from build123d import *

# Parameters (mm, degrees)
SKETCH1_R           = 5.9375
SKETCH1_R_2         = 1.4375
BOSS_EXTRUDE1_DEPTH = 6.35
SKETCH8_R           = 1.5
CUT_EXTRUDE1_DEPTH  = 45.18177233


with BuildPart() as part:
    # Sketch1 → Boss-Extrude1 (new body)
    with BuildSketch(Plane.XY):
        with BuildLine():
            ThreePointArc((7.766045394, -32.993333104), (18.228763262, -27.492050685), (19.627171546, -15.754204728))
            Line((19.627171546, -15.754204728), (11.861126152, 4.539128375))
            ThreePointArc((11.861126152, 4.539128375), (1.909586496, 12.555615453), (-9.975303898, 7.860236137))
            Line((-9.975303898, 7.860236137), (-25.965833293, -12.433096966))
            ThreePointArc((-25.965833293, -12.433096966), (-27.416705459, -25.837023258), (-15.990529394, -32.993333104))
            Line((-15.990529394, -32.993333104), (7.766045394, -32.993333104))
        make_face()
        with Locations((-15.990529394, -20.293333104)):
            Circle(SKETCH1_R, mode=Mode.SUBTRACT)
        with Locations((7.766045394, -20.293333104)):
            Circle(SKETCH1_R, mode=Mode.SUBTRACT)
        Circle(SKETCH1_R_2, mode=Mode.SUBTRACT)
    extrude(amount=BOSS_EXTRUDE1_DEPTH)

    # Sketch8 → Cut-Extrude1 (cut, through all)
    with BuildSketch(Plane.XY.offset(6.35)):
        with Locations((7.766045394, -10.768333104)):
            Circle(SKETCH8_R)
        with Locations((-15.990529394, -29.818333104)):
            Circle(SKETCH8_R)
        with Locations((-24.239421365, -15.530833104)):
            Circle(SKETCH8_R)
        with Locations((-7.741637423, -15.530833104)):
            Circle(SKETCH8_R)
        with Locations((16.014937365, -25.055833104)):
            Circle(SKETCH8_R)
        with Locations((-0.482846577, -25.055833104)):
            Circle(SKETCH8_R)
    extrude(amount=-CUT_EXTRUDE1_DEPTH, mode=Mode.SUBTRACT)


solid = part.part
The model under review builds one solid part; all positions refer to its coordinate system, in mm. Coordinates: 2 decimals unless noted, no trailing zeros. Write each loop counter-clockwise with the first axis right and the second up, starting at its lowest first coordinate (ties: lowest second). Pieces come first, ordered by that corner, then holes. Notation, with made-up numbers: (-15.75, 50.5) -> (17.25, 50.5) arc R16 cw to (17.25, 63.5) -> close; hole circle Ø6 at (8.5, 77.5). An arc over 180 degrees is marked (long way). Answer in a Markdown table with one row per item.
1. Clearance check with flat-ended pins moving along their axes: pin 1 Ø10.5 at (x, y) = (-15.99, -20.29) entering from +Z; pin 2 Ø3 at (y, z) = (-2.5, 3) entering from -X. State where each tip first meets the part, or that it passes through.
Answers below:
| item | result |
|---|---|
| pin 1 | passes through |
| pin 2 | stops at x = -19.32 |
2. Draft analysis for pull direction X (two halves, no side actions). For faces 1 (the flat face through (15.8, -5.75, 3.13)), 2 (the cylindrical face through (15.69, -26.52, 3.22)), 3 (the cylindrical face through (-0.81, -26.52, 3.22)), 4 (the cylindrical face through (2.095, 12.526, 3.131)), state which applies: +X half, -X half, draft (parallel to the pull), parting line (faces both ways), or undercut.
Answers below:
| item | result |
|---|---|
| face 1 | +X half |
| face 2 | undercut |
| face 3 | undercut |
| face 4 | parting line |
3. We need section A-A, the plane x = 10. State the section outline as (y, z) points, and give its area (3 significant figures).
Answers below:
| item | result |
|---|---|
| outline | (-32.8, 0) -> (-25.79, 0) -> (-25.79, 6.35) -> (-32.8, 6.35) -> close; (-14.79, 0) -> (7.83, 0) -> (7.83, 6.35) -> (-14.79, 6.35) -> close |
| area | 188 mm^2 |
4. We need section C-C, the plane x = 0. State the section outline as (y, z) points, and give its area (3 significant figures).
Answers below:
| item | result |
|---|---|
| outline | (-32.99, 0) -> (-26.48, 0) -> (-26.48, 6.35) -> (-32.99, 6.35) -> close; (-23.64, 0) -> (-1.44, 0) -> (-1.44, 6.35) -> (-23.64, 6.35) -> close; (1.44, 0) -> (12.7, 0) -> (12.7, 6.35) -> (1.44, 6.35) -> close |
| area | 254 mm^2 |
5. We need section B-B, the plane y = 0. State the section outline as (x, z) points, and give its area (3 significant figures).
Answers below:
| item | result |
|---|---|
| outline | (-16.17, 0) -> (-1.44, 0) -> (-1.44, 6.35) -> (-16.17, 6.35) -> close; (1.44, 0) -> (13.6, 0) -> (13.6, 6.35) -> (1.44, 6.35) -> close |
| area | 171 mm^2 |
6. We need section D-D, the plane y = -18. State the section outline as (x, z) points.
Answers below:
| item | result |
|---|---|
| outline | (-28.48, 0) -> (-21.47, 0) -> (-21.47, 6.35) -> (-28.48, 6.35) -> close; (-10.51, 0) -> (2.29, 0) -> (2.29, 6.35) -> (-10.51, 6.35) -> close; (13.24, 0) -> (20.26, 0) -> (20.26, 6.35) -> (13.24, 6.35) -> close |
7. Wall thickness on probe 1 along X at (y, z) = (-15, 4.75); probe 2 along Y at (x, z) = (0, 2.25); probe 3 along X at (y, z) = (-18, 2.5): over which ranges is each line inside the solid? List them lowest first. Write a range as [from, to].
Answers below:
| item | result |
|---|---|
| probe 1 | x = [-27.53, -25.64], [-22.84, -18.68], [-13.3, -9.14], [-6.34, 5.08], [10.46, 19.34] |
| probe 2 | y = [-32.99, -26.48], [-23.64, -1.44], [1.44, 12.7] |
| probe 3 | x = [-28.48, -21.47], [-10.51, 2.29], [13.24, 20.26] |
